For this review, take the finished solid that the model builds, in its own axes (mm). A direction names the side the tool comes from. Coordinates: 2 decimals unless noted, no trailing zeros. Order: outer loops, then holes, each group sorted by start corner. A loop starts at its lowest first (then second) coordinate and runs counter-clockwise, first axis right, second up.
from build123d import *

# Parameters (mm, degrees)
SKETCH1_W                      = 50
SKETCH1_H                      = 50
BOSS_EXTRUDE1_DEPTH            = 20
FILLET1_R                      = 5
CUT_EXTRUDE1_REACH             = 75.485
SKETCH2_R                      = 5
BOSS_EXTRUDE2_DEPTH            = 40
BOSS_EXTRUDE2_DEPTH_BACK       = 40
SKETCH3_W                      = 10
SKETCH3_H                      = 50
M3_CLEARANCE_HOLE1_D           = 3.4
M3_CLEARANCE_HOLE1_CSINK_D     = 3.45
M3_CLEARANCE_HOLE1_CSINK_ANGLE = 90


with BuildPart() as part:
    # Sketch1 → Boss-Extrude1 (new body)
    with BuildSketch(Plane(origin=(0, 0, 0), x_dir=(1, 0, 0), z_dir=(0, 1, 0))):
        with Locations((25, 0)):
            Rectangle(SKETCH1_W, SKETCH1_H)
    extrude(amount=BOSS_EXTRUDE1_DEPTH)

    # Fillet1
    fillet1_edges = [part.edges().sort_by_distance(p)[0] for p in [
        (50, 10, -25),
        (50, 10, 25),
    ]]
    fillet(fillet1_edges, radius=FILLET1_R)

    # Sketch2 → Cut-Extrude1 (cut, up to next)
    with BuildSketch(Plane.XY.offset(25), mode=Mode.PRIVATE) as cut_extrude1_sk1:
        with Locations((40, 10)):
            Circle(SKETCH2_R)
    cut_extrude1_tool1 = extrude(cut_extrude1_sk1.sketch, amount=-CUT_EXTRUDE1_REACH, mode=Mode.PRIVATE) & part.part
    add(cut_extrude1_tool1.solids().sort_by_distance((40, 10, 25))[0], mode=Mode.SUBTRACT)

    # Sketch3 → Boss-Extrude2 (add, two sides: drawn at the far end of the back side and taken through both)
    with BuildSketch(Plane(origin=(0, 10, 0), x_dir=(1, 0, 0), z_dir=(0, 1, 0)).offset(-BOSS_EXTRUDE2_DEPTH_BACK)):
        with Locations((5, 0)):
            Rectangle(SKETCH3_W, SKETCH3_H)
    extrude(amount=BOSS_EXTRUDE2_DEPTH + BOSS_EXTRUDE2_DEPTH_BACK)

    # M3 Clearance Hole1 (through all)
    with Locations(Plane.ZY):
        with Locations((-19, 44), (19, 44), (-19, -24), (19, -24)):
            CounterSinkHole(M3_CLEARANCE_HOLE1_D / 2, M3_CLEARANCE_HOLE1_CSINK_D / 2, counter_sink_angle=M3_CLEARANCE_HOLE1_CSINK_ANGLE)


solid = part.part
1. Clearance check with flat-ended pins moving along their axes: pin 1 Ø15 at (y, z) = (30, -6.5) entering from +X; pin 2 Ø10 at (x, z) = (32, 14) entering from +Y; pin 3 Ø6 at (x, z) = (41, 2.5) entering from -Y. State where each tip first meets the part, or that it passes through.
Answer below:
pin 1: stops at x = 10
pin 2: stops at y = 20
pin 3: stops at y = 0
2. Take a section at B-B, the plane y = 44. Give the boundary of the cut face in (x, z) (3 decimals).
Answer below:
outline: (0, -25) - (10, -25) - (10, -20.7) - (0.025, -20.7) - (0, -20.725) - close; (0, -17.275) - (0.025, -17.3) - (10, -17.3) - (10, 17.3) - (0.025, 17.3) - (0, 17.275) - close; (0, 20.725) - (0.025, 20.7) - (10, 20.7) - (10, 25) - (0, 25) - close
3. To check wall thickness, follow L1, parallel to Y at x = 2, z = -19; L2, parallel to Z at x = 2, y = -24; L3, parallel to Y at x = 40, z = -9. State the ranges of each line that lie inside material, in increasing order.
Answer below:
L1: y = -30 to -25.7, -22.3 to 42.3, 45.7 to 50
L2: z = -25 to -20.7, -17.3 to 17.3, 20.7 to 25
L3: y = 0 to 5, 15 to 20
4. Take a section at C-C, the plane z = -11. Give the boundary of the cut face in (x, y), plus the area to 3 significant figures.
Answer below:
outline: (0, -30) - (10, -30) - (10, 0) - (50, 0) - (50, 20) - (10, 20) - (10, 50) - (0, 50) - close; hole circle Ø10 at (40, 10)
area: 1,520 mm2
5. Take a section at D-D, the plane y = 8.5. Give the boundary of the cut face in (x, z).
Answer below:
outline: (0, -25) - (35.23, -25) - (35.23, 25) - (0, 25) - close; (44.77, -25) - (45, -25) arc R5 ccw to (50, -20) - (50, 20) arc R5 ccw to (45, 25) - (44.77, 25) - close
6. The part is to be moulded in two halves that separate along Y. For faces 4 (the face through (5, -30, 0)), 5 (the face through (49, 10, -23)), 6 (the face through (30, 20, 0)), 7 (the face through (5.1, 42.5, -19.8)), say which applies: +Y half, -Y half, draft (parallel to the pull), parting line (faces both ways), or undercut.
Answer below:
face 4: -Y half
face 5: draft
face 6: +Y half
face 7: undercut
7. Machinability: for faces 1 (the face through (10, -15, 0)), 2 (the face through (5, 50, 0)), 3 (the face through (10, 35, 0)), which of the approach directions +Z, -Z, +X, -X, +Y, -Y give a long, thin tool a straight path to every point of the face, cutting with its end or side? Answer none if there is none.
Answer below:
face 1: +Z, -Z, +X, -Y
face 2: +Z, -Z, +X, -X, +Y
face 3: +Z, -Z, +X, +Y
8. Take a section at A-A, the plane z = 19. Give the boundary of the cut face in (x, y) (3 decimals), plus the area to 3 significant figures.
Answer below:
outline: (0, -30) - (10, -30) - (10, -25.7) - (0.025, -25.7) - (0, -25.725) - close; (0, -22.275) - (0.025, -22.3) - (10, -22.3) - (10, 0) - (50, 0) - (50, 20) - (10, 20) - (10, 42.3) - (0.025, 42.3) - (0, 42.275) - close; (0, 45.725) - (0.025, 45.7) - (10, 45.7) - (10, 50) - (0, 50) - close; hole circle Ø10 at (40, 10)
area: 1,450 mm2
